Could you check a few things on this model? Use its own coordinates, in mm. Round coordinates to 2 decimals unless told otherwise and drop trailing zeros. Write each loop counter-clockwise with the first axis right and the second up, starting at its lowest first coordinate (ties: lowest second). Pieces come first, ordered by that corner, then holes. Notation, with made-up numbers: M 14.5,10 L 46.5,10 A28 cw 46.5,36 Z; hole C 1,79.5 d1. An arc over 180 degrees is marked long. One line per item, written item: value. Start each with the question number.
(1) I'm going to push flat-ended pins straight in: pin 1 Ø5 at (x, z) = (0, 3.81) entering from -Y; pin 2 Ø3 at (x, y) = (2, -2.5) entering from -Z; pin 3 Ø6 at (x, z) = (-4, 4.5) entering from +Y. Where does each tip first touch, or does it pass through?
(2) I want a section at C-C on x = -1. Count the separate pieces of the cut face and the enclosed holes in it, and give its area (3 significant figures).
(3) Thinking about a two-plate mould opening in Y: for faces 1 (the face through (-1.83, 3.53, 4.54)), 2 (the face through (-3.536, -0.07, 10.587)), 3 (the face through (5.13, -2.13, 5.63)), 4 (the face through (-0.548, 0.42, 9.746)), which applies, released by +Y, released by -Y, zero draft, split by the parting line, or undercut?
(4) I want a section at B-B on z = 1.75. Please give me the cut outline in (x, y), and give its area (3 significant figures).
(5) I want a section at A-A on z = 3.81. Please give me the cut outline in (x, y).
(6) If I drill on L1, parallel to X at y = 4.55, z = 3.81; L2, parallel to X at y = 1.75, z = 6.25; L3, parallel to Y at x = 3, z = 5, over which ranges is the centre line in solid material (lowest first)?
(7) I want a section at D-D on z = 8. Please give me the cut outline in (x, y).
```python
from build123d import *

# Parameters (mm, degrees)
F0_R     = 5.55625
F1_DEPTH = 11.43
F3_D     = 7.9502
F3_DEPTH = 7.7724
F3_TIP   = 2.3884810467
F4_R     = 6.35
F5_DEPTH = 12.7
F6_R     = 1.6002
F7_DEPTH = 12.7


with BuildPart() as f1:
    # F0 (on Top) → F1 (new body)
    with BuildSketch(Plane.XY):
        Circle(F0_R)
    extrude(amount=F1_DEPTH)

    # F3
    with Locations(Plane(origin=(0, 0, 0), x_dir=(1, 0, 0), z_dir=(0, 0, -1))):
        with Locations((0, 0)):
            Hole(F3_D / 2, depth=F3_DEPTH)
            with Locations((0, 0, -(F3_DEPTH + F3_TIP / 2))):  # 118° drill point
                Cone(0, F3_D / 2, F3_TIP, mode=Mode.SUBTRACT)

    # F4 (on Front) → F5 (cut, symmetric)
    with BuildSketch(Plane.XZ):
        with Locations((-6.72465, 16.0782)):
            Circle(F4_R)
    extrude(amount=F5_DEPTH, both=True, mode=Mode.SUBTRACT)

    # F6 (on Front) → F7 (cut, symmetric)
    with BuildSketch(Plane.XZ):
        with Locations((0, 3.81)):
            Circle(F6_R)
    extrude(amount=F7_DEPTH, both=True, mode=Mode.SUBTRACT)

    # F8 (on Front) → F9 (revolve, cut)
    with BuildSketch(Plane.XZ):
        Polygon((-3.9751, 0), (-3.9751, 1.209802), (-5.184902, 0), align=None)
    revolve(axis=Axis((0, 0, 6.5590362065), (0, 0, 1)), mode=Mode.SUBTRACT)


solid = f1.part
```
Found:
1. pin 1: stops at y = -5.56
1. pin 2: stops at z = 0.48
1. pin 3: stops at y = 5.46
2. separate pieces: 3
2. enclosed holes: 0
2. area: 47.6 mm²
3. face 1: undercut
3. face 2: zero draft
3. face 3: split by the parting line
3. face 4: undercut
4. outline: C 0,0 d11.11; hole C 0,0 d7.95
4. area: 47.3 mm²
5. outline: M -1.6,-5.32 L -1.6,-3.64 A3.98 cw -1.6,3.64 L -1.6,5.32 A5.56 ccw Z; M 1.6,-5.32 A5.56 ccw 1.6,5.32 L 1.6,3.64 A3.98 cw 1.6,-3.64 Z
6. L1: x = -3.19 to -1.6, 1.6 to 3.19
6. L2: x = -5.27 to -3.57, 3.57 to 5.27
6. L3: y = -4.68 to -2.61, 2.61 to 4.68
7. outline: C 0,0 d11.11; hole C 0,0 d7.19
